The model under review builds one solid part; all positions refer to its coordinate system, in mm. A direction names the side the tool comes from. Round coordinates to 2 decimals unless told otherwise and drop trailing zeros. Order: outer loops, then holes, each group sorted by start corner. A loop starts at its lowest first (then second) coordinate and runs counter-clockwise, first axis right, second up. Notation, with made-up numbers: (15, 19) -> (54, 19) arc R20 ccw to (54, 57) -> close; hole circle Ø4 at (79, 11). An arc over 180 degrees is marked (long way). Use a Markdown table: item, result. Add a question column.
```python
from build123d import *

# Parameters (mm, degrees)
SKETCH2_R           = 5.0038
BOSS_EXTRUDE1_DEPTH = 5
SKETCH3_R           = 6
BOSS_EXTRUDE2_DEPTH = 5
SKETCH5_R           = 6
BOSS_EXTRUDE3_DEPTH = 5
SKETCH6_R           = 5
BOSS_EXTRUDE4_DEPTH = 5
SKETCH8_R           = 2.698107805
BOSS_EXTRUDE5_DEPTH = 4.6
CUT_EXTRUDE1_DEPTH  = 1


with BuildPart() as part:
    # Sketch2 → Boss-Extrude1 (new body)
    with BuildSketch(Plane.XY.offset(-1161.582265199)):
        Circle(SKETCH2_R)
        with BuildLine():
            Line((2, 1.5), (2, -1.5))
            ThreePointArc((2, -1.5), (-2.5, 0), (2, 1.5))
        make_face(mode=Mode.SUBTRACT)
    extrude(amount=BOSS_EXTRUDE1_DEPTH)

    # Sketch3 → Boss-Extrude2 (add)
    with BuildSketch(Plane.XY.offset(-1156.582265199)):
        with Locations(Location((1.25, 0, 0), (0, 0, 213.387732771))):
            Circle(SKETCH3_R)
        with BuildLine():
            Line((2, 1.5), (2, -1.5))
            ThreePointArc((2, -1.5), (-2.5, 0), (2, 1.5))
        make_face(mode=Mode.SUBTRACT)
    extrude(amount=BOSS_EXTRUDE2_DEPTH)

    # Sketch5 → Boss-Extrude3 (add)
    with BuildSketch(Plane.XY.offset(-1151.582265199)):
        with Locations(Location((-1.25, 0, 0), (0, 0, 282.024699181))):
            Circle(SKETCH5_R)
        with BuildLine():
            Line((2, 1.5), (2, -1.5))
            ThreePointArc((2, -1.5), (-2.5, 0), (2, 1.5))
        make_face(mode=Mode.SUBTRACT)
    extrude(amount=BOSS_EXTRUDE3_DEPTH)

    # Sketch6 → Boss-Extrude4 (add)
    with BuildSketch(Plane.XY.offset(-1146.582265199)):
        with Locations(Location((0, 0, 0), (0, 0, 319.025369771))):
            Circle(SKETCH6_R)
        with BuildLine():
            Line((2, 1.5), (2, -1.5))
            ThreePointArc((2, -1.5), (-2.5, 0), (2, 1.5))
        make_face(mode=Mode.SUBTRACT)
    extrude(amount=BOSS_EXTRUDE4_DEPTH)

    # Sketch8 → Boss-Extrude5 (add)
    with BuildSketch(Plane.XY.offset(-1146.182265199)):
        Circle(SKETCH8_R)
    extrude(amount=BOSS_EXTRUDE5_DEPTH)

    # Sketch9 → Cut-Extrude1 (cut)
    with BuildSketch(Plane.XY.offset(-1141.582265199)):
        Polygon((0, 4.107590662), (-3.557277862, -2.053795331), (3.557277862, -2.053795331), align=None)
        Polygon((0, 3.010552133), (-2.607214626, -1.505276066), (2.607214626, -1.505276066), align=None, mode=Mode.SUBTRACT)
    extrude(amount=-CUT_EXTRUDE1_DEPTH, mode=Mode.SUBTRACT)


solid = part.part
```
Q1. Add section B-B, the plane y = 2.25. Give the boundary of the cut face in (x, z).
Q2. Add section A-A, the plane z = -1160.25. Give the boundary of the cut face in (x, y).
Q3. For pin 1 (3 mm diameter, centred on x = 5, z = -1149.5, fed in from -Y); pin 2 (1.3 mm diameter, centred on x = 0, y = 1, fed in from -Z); pin 3 (3.5 mm diameter, centred on y = 0, z = -1157.5, fed in from -X), all flat-tipped, find the tip position at first contact; note any pin that passes through.
Q4. Add section C-C, the plane x = -4.25. Give the boundary of the cut face in (y, z), then the cut area to 3 significant figures.
Q5. For faces 1 (the face through (1.322, 0.721, -1142.075)), 2 (the face through (-2.54, -4.65, -1154.12)), 3 (the face through (2, 0, -1154)), list the 3-axis set-ups (+Z, -Z, +X, -X, +Y, -Y) from which the entire face can be reached by the end or side of a thin tool; tool diameter is ignored.
Q6. To check wall thickness, follow line 1 along Y through (x, z) = (0, -1157.5); line 2 along X through (y, z) = (0, -1156); line 3 along Z through (x, y) = (-4.75, -1). State the ranges of each line that lie inside material, in increasing order.
Q7. Draft analysis for pull direction Y (two halves, no side actions). For faces 4 (the face through (0, 0, -1146.182)), 5 (the face through (-7.25, 0.05, -1149.12)), 6 (the face through (2.2, 0.1, -1161.582)), state which applies: released by +Y, released by -Y, zero draft, split by the parting line, or undercut.
Q8. Add section D-D, the plane x = 1.25. Give the boundary of the cut face in (y, z), then the cut area to 3 significant figures.
Return value:
| question | item | result |
|---|---|---|
| 1 | outline | (-6.81, -1151.58) -> (-4.31, -1151.58) -> (-4.31, -1156.58) -> (-4.47, -1156.58) -> (-4.47, -1161.58) -> (-1.09, -1161.58) -> (-1.09, -1146.18) -> (1.09, -1146.18) -> (1.09, -1161.58) -> (4.47, -1161.58) -> (4.47, -1156.58) -> (6.81, -1156.58) -> (6.81, -1151.58) -> (4.31, -1151.58) -> (4.31, -1146.58) -> (4.47, -1146.58) -> (4.47, -1141.58) -> (1.07, -1141.58) -> (1.07, -1142.58) -> (0.44, -1142.58) -> (0.44, -1141.58) -> (-0.44, -1141.58) -> (-0.44, -1142.58) -> (-1.07, -1142.58) -> (-1.07, -1141.58) -> (-4.47, -1141.58) -> (-4.47, -1146.58) -> (-6.81, -1146.58) -> close |
| 2 | outline | circle Ø10.01 at (0, 0); hole (2, -1.5) -> (2, 1.5) arc R2.5 ccw (long way) to start |
| 3 | pin 1 | y = -3.67 |
| 3 | pin 2 | z = -1146.18 |
| 3 | pin 3 | x = -5 |
| 4 | outline | (-5.2, -1151.58) -> (-2.4, -1151.58) -> (-2.4, -1156.58) -> (-2.64, -1156.58) -> (-2.64, -1161.58) -> (2.64, -1161.58) -> (2.64, -1156.58) -> (2.4, -1156.58) -> (2.4, -1151.58) -> (5.2, -1151.58) -> (5.2, -1146.58) -> (2.63, -1146.58) -> (2.63, -1141.58) -> (-2.63, -1141.58) -> (-2.63, -1146.58) -> (-5.2, -1146.58) -> close |
| 4 | area | 129 mm² |
| 5 | face 1 | +Z |
| 5 | face 2 | none |
| 5 | face 3 | -Z |
| 6 | line 1 | -5 to -2.5, 2.5 to 5 |
| 6 | line 2 | -4.75 to -2.5, 2 to 7.25 |
| 6 | line 3 | -1161.58 to -1156.58, -1151.58 to -1141.58 |
| 7 | face 4 | undercut |
| 7 | face 5 | split by the parting line |
| 7 | face 6 | zero draft |
| 8 | outline | (-6, -1156.58) -> (-4.85, -1156.58) -> (-4.85, -1161.58) -> (-2.17, -1161.58) -> (-2.17, -1146.18) -> (2.17, -1146.18) -> (2.17, -1161.58) -> (4.85, -1161.58) -> (4.85, -1156.58) -> (6, -1156.58) -> (6, -1151.58) -> (5.45, -1151.58) -> (5.45, -1146.58) -> (4.84, -1146.58) -> (4.84, -1141.58) -> (1.94, -1141.58) -> (1.94, -1142.58) -> (0.85, -1142.58) -> (0.85, -1141.58) -> (-1.51, -1141.58) -> (-1.51, -1142.58) -> (-2.05, -1142.58) -> (-2.05, -1141.58) -> (-4.84, -1141.58) -> (-4.84, -1146.58) -> (-5.45, -1146.58) -> (-5.45, -1151.58) -> (-6, -1151.58) -> close |
| 8 | area | 143 mm² |
